from build123d import *

# Parameters (mm, degrees)
F1_DEPTH = 114
F3_DEPTH = 82


with BuildPart() as f1:
    # F0 (on Top) → F1 (new body)
    with BuildSketch(Plane.XY):
        Polygon((-56.6203880661, 9.7190998064), (25.3796119339, 9.7190998064), (12.379645281, 12.2834371362), (-15.6203880661, 12.22001634), (-43.6204214132, 12.2834371362), align=None)
        Polygon((-15.6203880661, -0.7809001936), (25.3796119339, -0.7809001936), (25.3796119339, 9.7190998064), (-56.6203880661, 9.7190998064), (-56.6203880661, -0.7809001936), align=None)
        Polygon((25.3796119339, -11.2809001936), (25.3796119339, -0.7809001936), (-15.6203880661, -0.7809001936), (-56.6203880661, -0.7809001936), (-56.6203880661, -11.2809001936), align=None)
        Polygon((12.379645281, -13.8452375234), (25.3796119339, -11.2809001936), (-56.6203880661, -11.2809001936), (-43.6204214132, -13.8452375234), (-15.6203880661, -13.7818167272), align=None)
    extrude(amount=F1_DEPTH)

    # F2 (on face) → F3 (join)
    with BuildSketch(Plane.YZ.offset(25.3796119339)):
        with BuildLine():
            ThreePointArc((-11.2809001936, 131.8843561195), (-12.5, 126.5), (-11.2809001936, 121.1156438805))
            Line((-11.2809001936, 121.1156438805), (-11.2809001936, 131.8843561195))
        make_face()
        with BuildLine():
            Line((-11.2809001936, 114), (0, 114))
            ThreePointArc((0, 114), (-6.6687910638, 115.9275250888), (-11.2809001936, 121.1156438805))
            Line((-11.2809001936, 121.1156438805), (-11.2809001936, 114))
        make_face()
        with BuildLine():
            ThreePointArc((-11.2809001936, 121.1156438805), (-6.6687910638, 115.9275250888), (0, 114))
            Line((0, 114), (0, 116.5))
            ThreePointArc((0, 116.5), (-9.4868329805, 123.3377223398), (-6, 134.5))
            Line((-6, 134.5), (-6, 137.4658560997))
            ThreePointArc((-6, 137.4658560997), (-9.0799594373, 135.0909450363), (-11.2809001936, 131.8843561195))
            Line((-11.2809001936, 131.8843561195), (-11.2809001936, 121.1156438805))
        make_face()
        with BuildLine():
            Line((0, 116.5), (0, 114))
            ThreePointArc((0, 114), (6.6687910638, 115.9275250888), (11.2809001936, 121.1156438805))
            Line((11.2809001936, 121.1156438805), (11.2809001936, 131.8843561195))
            ThreePointArc((11.2809001936, 131.8843561195), (9.0799594373, 135.0909450363), (6, 137.4658560997))
            Line((6, 137.4658560997), (6, 134.5))
            ThreePointArc((6, 134.5), (8.94427191, 130.972135955), (10, 126.5))
            ThreePointArc((10, 126.5), (7.0710678119, 119.4289321881), (0, 116.5))
        make_face()
        with BuildLine():
            ThreePointArc((11.2809001936, 121.1156438805), (6.6687910638, 115.9275250888), (0, 114))
            Line((0, 114), (9.7190998064, 114))
            Line((9.7190998064, 114), (11.2809001936, 114))
            Line((11.2809001936, 114), (11.2809001936, 121.1156438805))
        make_face()
        with BuildLine():
            Line((11.2809001936, 131.8843561195), (11.2809001936, 121.1156438805))
            ThreePointArc((11.2809001936, 121.1156438805), (12.1914160872, 123.7396786799), (12.5, 126.5))
            ThreePointArc((12.5, 126.5), (12.1914160872, 129.2603213201), (11.2809001936, 131.8843561195))
        make_face()
    extrude(amount=-F3_DEPTH)


solid = f1.part
For this review, take the finished solid that the model builds, in its own axes (mm). A direction names the side the tool comes from. Coordinates: 2 decimals unless noted, no trailing zeros. Loops run counter-clockwise (first coordinate to the right, second up) from the corner with the lowest first, then second, coordinate; pieces in that order, holes last. Notation, with made-up numbers: (8, 27) - (67, 27) arc R15 ccw to (67, 55) - close; hole circle Ø5 at (79, 14). An arc over 180 degrees is marked (long way). Use a Markdown table: item, result. Add a question column.
Item 1: Mouldability with a two-part tool opening along Z and no side actions: class faces 1 (the face through (-15, -11.281, 118)), 2 (the face through (25.38, 0, 70)), 3 (the face through (-16, -1, 0)) as pulls with the +Z half, pulls with the -Z half, needs draft (parallel to the pull), parting line crosses it, or undercut.
Item 2: For line 1 (Y direction, x = -43, z = 87); line 2 (Y direction, x = -5, z = 103); line 3 (Z direction, x = 2, y = -8.75), list the stretches that pass through material, from the lowest coordinate up.
Item 3: Tool access review of faces 4 (the face through (-15, 11.281, 118)), 5 (the face through (-50.03, 11.02, 56.2)), 6 (the face through (-16, -13, 114)), 7 (the face through (18.79, -12.58, 56.2)): name each direction out of +Z, -Z, +X, -X, +Y, -Y from which nothing blocks a thin tool from reaching the whole face with its end or side.
Item 4: We need section A-A (z = 84). Give the boundary of the cut face in (x, y), and give its area (3 significant figures).
Item 5: We need section B-B (y = 7.75). Give the boundary of the cut face in (x, z), and give its area (3 significant figures).
Item 6: Insertion check: pin 1 Ø2.5 at (x, z) = (-23.5, 136.5) entering from +Y; pin 2 Ø3.5 at (x, z) = (-15, 136) entering from -Y; pin 3 Ø3 at (x, z) = (-26.5, 122) entering from -Y. Each pin has a flat end and moves straight along its axis. Give the tip position at first contact, or say it passes through.
Item 7: We need section D-D (x = -0.5). Give the boundary of the cut face in (y, z).
Item 8: We need section C-C (x = -18). Give the boundary of the cut face in (y, z), and give its area (3 significant figures).
Results list:
| question | item | result |
|---|---|---|
| 1 | face 1 | undercut |
| 1 | face 2 | needs draft |
| 1 | face 3 | pulls with the -Z half |
| 2 | line 1 | y = -13.84 to 12.28 |
| 2 | line 2 | y = -13.81 to 12.24 |
| 2 | line 3 | z = 0 to 121.66, 131.34 to 135.43 |
| 3 | face 4 | +X, -X, +Y |
| 3 | face 5 | -Z, -X, +Y |
| 3 | face 6 | +X, -X, -Y |
| 3 | face 7 | -Z, +X, -Y |
| 4 | outline | (-56.62, -11.28) - (-43.62, -13.85) - (-15.62, -13.78) - (12.38, -13.85) - (25.38, -11.28) - (25.38, 9.72) - (12.38, 12.28) - (-15.62, 12.22) - (-43.62, 12.28) - (-56.62, 9.72) - close |
| 4 | area | 2,070 mm^2 |
| 5 | outline | (-56.62, 0) - (25.38, 0) - (25.38, 120.18) - (-56.62, 120.18) - close; (-56.62, 132.82) - (25.38, 132.82) - (25.38, 136.31) - (-56.62, 136.31) - close |
| 5 | area | 10,100 mm^2 |
| 6 | pin 1 | stops at y = 8.93 |
| 6 | pin 2 | stops at y = -9.81 |
| 6 | pin 3 | stops at y = -12.13 |
| 7 | outline | (-13.82, 0) - (12.25, 0) - (12.25, 114) - (11.28, 114) - (11.28, 121.12) arc R12.5 ccw to (6, 137.47) - (6, 134.5) arc R10 cw (long way) to (-6, 134.5) - (-6, 137.47) arc R12.5 ccw to (-11.28, 121.12) - (-11.28, 114) - (-13.82, 114) - close |
| 8 | outline | (-13.79, 0) - (12.23, 0) - (12.23, 114) - (11.28, 114) - (11.28, 121.12) arc R12.5 ccw to (6, 137.47) - (6, 134.5) arc R10 cw (long way) to (-6, 134.5) - (-6, 137.47) arc R12.5 ccw to (-11.28, 121.12) - (-11.28, 114) - (-13.79, 114) - close |
| 8 | area | 3,160 mm^2 |
